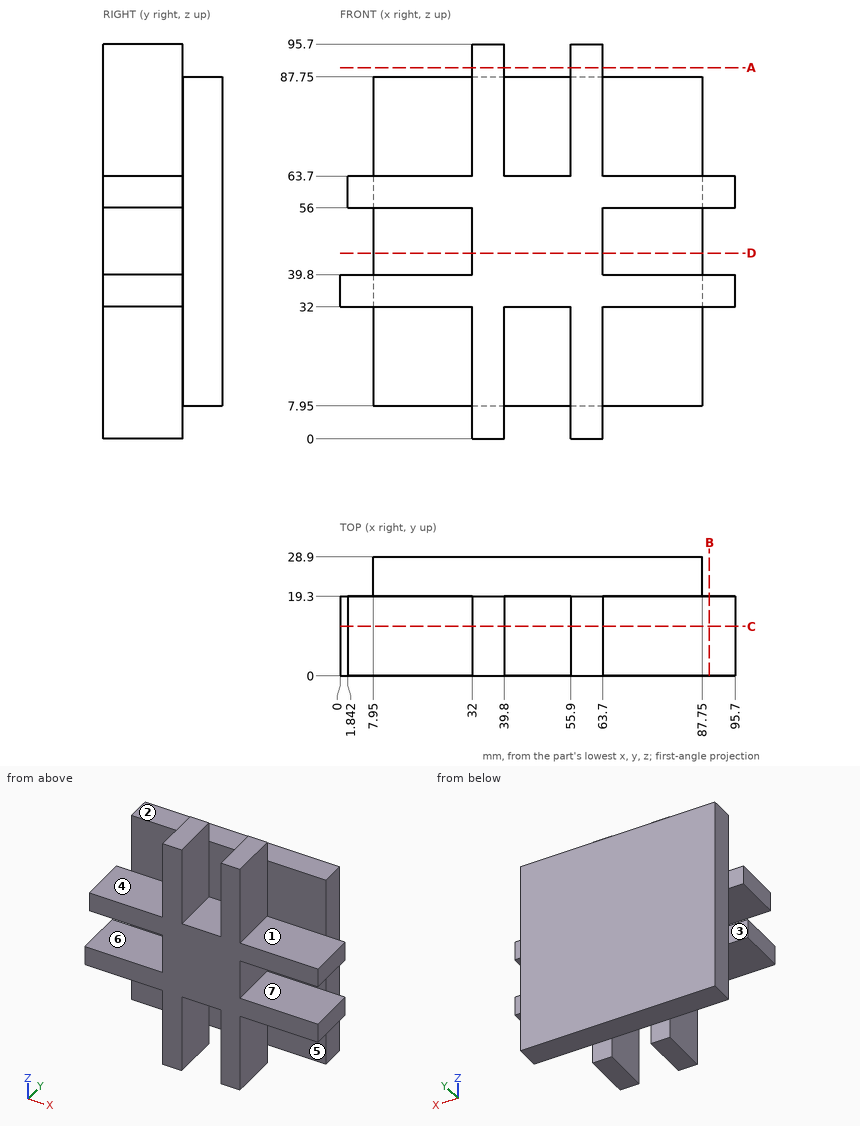
Part print with two shaded views. Sizes in mm from the minimum x, y, z corner. A direction names the side the tool comes from. Round coordinates to 2 decimals unless told otherwise and drop trailing zeros. Write each loop counter-clockwise with the first axis right and the second up, starting at its lowest first coordinate (ties: lowest second). Pieces come first, ordered by that corner, then holes. Notation, with made-up numbers: M 36,14.5 L 85,14.5 A30 cw 85,37.5 Z; hole C 2.5,8.5 d9. An arc over 180 degrees is marked long. Put each result on its own line as item: value. Start each with the question number.
1) 3-axis set-ups, long thin cutter, end or side, ignore diameter. For the marked faces 1, 2 and 3: which of +Z, -Z, +X, -X, +Y, -Y reach the whole face in a straight line?
2) Pull direction Z, two halves, no side cores. Call the marked faces 4, 5, 6 and 7: pulls with the +Z half, pulls with the -Z half, needs draft (parallel to the pull), parting line crosses it, or undercut.
3) Saw through at B-B, the plane x = 89.5. Write the cut outline in (y, z).
4) Saw through at D-D, the plane z = 45. Write the cut outline in (x, y), and give its area (3 significant figures).
5) Saw through at C-C, the plane y = 12. Write the cut outline in (x, z), and give its area (3 significant figures).
6) Pin check, flat tips, straight feed: pin 1 Ø15.5 at (x, y) = (21.5, 7) entering from +Z; pin 2 Ø7.5 at (x, y) = (46.5, 23.5) entering from +Z; pin 3 Ø10 at (y, z) = (3, 14.5) entering from -X. Stop position of each tip, or through.
7) Drill centre lines: probe 1 along Z at (x, y) = (5, 15); probe 2 along X at (y, z) = (6.75, 83.5); probe 3 along X at (y, z) = (22, 24.5). Where is each one in solid material? Low to high. Write a range as [from, to].
8) Saw through at A-A, the plane z = 90. Write the cut outline in (x, y).
Resolved:
1. face 1: +Z, +X, -Y
1. face 2: +Z, +X, -X, +Y
1. face 3: +Z, -Z, -X, +Y
2. face 4: pulls with the +Z half
2. face 5: needs draft
2. face 6: undercut
2. face 7: undercut
3. outline: M 0,32 L 19.3,32 L 19.3,39.8 L 0,39.8 Z; M 0,56 L 19.3,56 L 19.3,63.7 L 0,63.7 Z
4. outline: M 7.95,19.3 L 32,19.3 L 32,0 L 63.7,0 L 63.7,19.3 L 87.75,19.3 L 87.75,28.9 L 7.95,28.9 Z
4. area: 1,380 mm²
5. outline: M 0,32 L 32,32 L 32,0 L 39.8,0 L 39.8,32 L 55.9,32 L 55.9,0 L 63.7,0 L 63.7,32 L 95.7,32 L 95.7,39.8 L 63.7,39.8 L 63.7,56 L 95.7,56 L 95.7,63.7 L 63.7,63.7 L 63.7,95.7 L 55.9,95.7 L 55.9,63.7 L 39.8,63.7 L 39.8,95.7 L 32,95.7 L 32,63.7 L 1.84,63.7 L 1.84,56 L 32,56 L 32,39.8 L 0,39.8 Z
5. area: 2,980 mm²
6. pin 1: z = 63.7
6. pin 2: z = 87.75
6. pin 3: x = 32
7. probe 1: [32, 39.8], [56, 63.7]
7. probe 2: [32, 39.8], [55.9, 63.7]
7. probe 3: [7.95, 87.75]
8. outline: M 32,0 L 39.8,0 L 39.8,19.3 L 32,19.3 Z; M 55.9,0 L 63.7,0 L 63.7,19.3 L 55.9,19.3 Z
